```python
from build123d import *

# Parameters (mm, degrees)
F0_R     = 1.5
F0_R_2   = 1.75
F1_DEPTH = 2.5
F0_W     = 10
F0_H     = 10
F2_DEPTH = 100


# Not quite as in the source:
# - a feature names something its author has since deleted; it is built from what else it names


with BuildPart() as f1:
    # F0 (on Top) → F1 (new body)
    with BuildSketch(Plane.XY):
        Polygon((105.08390221, -67.8528748304), (85.08390221, -67.8528748304), (89.1031400965, -82.8528748304), (101.0646643235, -82.8528748304), align=None)
        with Locations((95.08390221, -78.8528748304)):
            Circle(F0_R, mode=Mode.SUBTRACT)
        Polygon((-47.91609779, 32.1471251696), (-57.91609779, 32.1471251696), (-57.91609779, -67.8528748304), (-47.91609779, -67.8528748304), (-27.91609779, -67.8528748304), (-17.91609779, -67.8528748304), (-17.91609779, -47.4599613249), (-27.91609779, -47.4599613249), (-27.91609779, -37.4599613249), (-17.91609779, -37.4599613249), (-17.91609779, 12.5400386751), (-27.91609779, 12.5400386751), (-27.91609779, 22.5400386751), (-17.91609779, 22.5400386751), (82.08390221, 22.5400386751), (97.08390221, 22.5400386751), (107.08390221, 22.5400386751), (107.08390221, 32.1471251696), (105.08390221, 32.1471251696), (85.08390221, 32.1471251696), (-27.91609779, 32.1471251696), align=None)
        with Locations((-37.91609779, -48.1028748304)):
            Circle(F0_R_2, mode=Mode.SUBTRACT)
        with Locations((-37.91609779, 16.8971251696)):
            Circle(F0_R_2, mode=Mode.SUBTRACT)
        Polygon((-27.91609779, -67.8528748304), (-47.91609779, -67.8528748304), (-43.8968599035, -82.8528748304), (-31.9353356765, -82.8528748304), align=None)
        with Locations((-37.91609779, -78.8528748304)):
            Circle(F0_R, mode=Mode.SUBTRACT)
        Polygon((-43.8968599035, 47.1471251696), (-47.91609779, 32.1471251696), (-27.91609779, 32.1471251696), (-31.9353356765, 47.1471251696), align=None)
        with Locations((-37.91609779, 43.1471251696)):
            Circle(F0_R, mode=Mode.SUBTRACT)
        Polygon((89.1031400965, 47.1471251696), (85.08390221, 32.1471251696), (105.08390221, 32.1471251696), (101.0646643235, 47.1471251696), align=None)
        with Locations((95.08390221, 43.1471251696)):
            Circle(F0_R, mode=Mode.SUBTRACT)
        Polygon((82.08390221, 12.5400386751), (82.08390221, -67.8528748304), (85.08390221, -67.8528748304), (105.08390221, -67.8528748304), (107.08390221, -67.8528748304), (107.08390221, -47.4599613249), (97.08390221, -47.4599613249), (97.08390221, -37.4599613249), (107.08390221, -37.4599613249), (107.08390221, 12.5400386751), (97.08390221, 12.5400386751), (97.08390221, 22.5400386751), (82.08390221, 22.5400386751), align=None)
        with Locations((88.28390221, -48.1028748304)):
            Circle(F0_R_2, mode=Mode.SUBTRACT)
        with Locations((88.28390221, 16.8971251696)):
            Circle(F0_R_2, mode=Mode.SUBTRACT)
    extrude(amount=F1_DEPTH)

    # F0 (on Top) → F2 (join)
    with BuildSketch(Plane.XY):
        with Locations((-22.91609779, 17.5400386751)):
            Rectangle(F0_W, F0_H)
        with Locations((102.08390221, 17.5400386751)):
            Rectangle(F0_W, F0_H)
        with Locations((102.08390221, -42.4599613249)):
            Rectangle(F0_W, F0_H)
        with Locations((-22.91609779, -42.4599613249)):
            Rectangle(F0_W, F0_H)
    extrude(amount=F2_DEPTH)


solid = f1.part
```
Part model, mm, in its own coordinate system. A direction names the side the tool comes from. Round coordinates to 2 decimals unless told otherwise and drop trailing zeros. Order: outer loops, then holes, each group sorted by start corner. A loop starts at its lowest first (then second) coordinate and runs counter-clockwise, first axis right, second up. Notation, with made-up numbers: M 29.25,83 L 50.25,83 A28 ccw 50.25,110 Z; hole C 76.25,64 d6. An arc over 180 degrees is marked long. Put each result on its own line as item: value. Start each with the question number.
1. Tool access for faces 5 (the face through (102, 12.54, 51)), 6 (the face through (102, 22.54, 51)), 7 (the face through (87, -75, 1)): list every direction of +Z, -Z, +X, -X, +Y, -Y with a clear straight run to the whole face (end or side of a thin tool).
2. Slice it at B-B on y = -19. List the corners of the cut face in (x, z).
3. Two-plate mould, pull along X, no slides. Class faces 1 (the face through (102, 18, 100)), 2 (the face through (87.12, 39.75, 1.23)), 3 (the face through (-27.916, -43, 51)), 4 (the face through (97.084, -43, 51)): +X half, -X half, draft (parallel to the pull), parting line (faces both ways), or undercut.
4. Slice it at D-D on y = 35. List the corners of the cut face in (x, z).
5. Drill centre lines: probe 1 along X at (y, z) = (-39, 34); probe 2 along Z at (x, y) = (95.5, -47.5). Where is each one in solid material? Low to high. Write a range as [from, to].
6. Slice it at C-C on x = -24. List the corners of the cut face in (y, z), then the cut area to 3 significant figures.
7. Drop flat-ended pins along their axis: pin 1 (0.8 mm diameter, centred on x = 45.5, z = 1.5, fed in from -Y); pin 2 (11 mm diameter, centred on x = -21, z = 52.5, fed in from -Y); pin 3 (11 mm diameter, centred on x = 103, z = 47, fed in from +Y). Give the stop position or say it passes through.
8. Slice it at A-A on z = 55.5. List the corners of the cut face in (x, y), then the cut area to 3 significant figures.
Findings:
1. face 5: +Z, +X, -X
1. face 6: +Z, +X, -X, +Y
1. face 7: +Z, -Z, -Y
2. outline: M -57.92,0 L -17.92,0 L -17.92,2.5 L -57.92,2.5 Z; M 82.08,0 L 107.08,0 L 107.08,2.5 L 82.08,2.5 Z
3. face 1: draft
3. face 2: undercut
3. face 3: -X half
3. face 4: undercut
4. outline: M -47.15,0 L -28.68,0 L -28.68,2.5 L -47.15,2.5 Z; M 85.85,0 L 104.32,0 L 104.32,2.5 L 85.85,2.5 Z
5. probe 1: [-27.92, -17.92], [97.08, 107.08]
5. probe 2: [0, 2.5]
6. outline: M -67.85,0 L 32.15,0 L 32.15,2.5 L 22.54,2.5 L 22.54,100 L 12.54,100 L 12.54,2.5 L -37.46,2.5 L -37.46,100 L -47.46,100 L -47.46,2.5 L -67.85,2.5 Z
6. area: 2,200 mm2
7. pin 1: y = 22.54
7. pin 2: y = -47.46
7. pin 3: y = 22.54
8. outline: M -27.92,-47.46 L -17.92,-47.46 L -17.92,-37.46 L -27.92,-37.46 Z; M -27.92,12.54 L -17.92,12.54 L -17.92,22.54 L -27.92,22.54 Z; M 97.08,-47.46 L 107.08,-47.46 L 107.08,-37.46 L 97.08,-37.46 Z; M 97.08,12.54 L 107.08,12.54 L 107.08,22.54 L 97.08,22.54 Z
8. area: 400 mm2
